from build123d import *

# Parameters (mm, degrees)
CSK_FOR_M3_FLAT_HEAD_MACHINE_SCREW1_AT_2_COUNT = 2
CSK_FOR_M3_FLAT_HEAD_MACHINE_SCREW1_AT_2_PITCH = 13.856406461
CSK_FOR_M3_FLAT_HEAD_MACHINE_SCREW1_AT_3_COUNT = 2
CSK_FOR_M3_FLAT_HEAD_MACHINE_SCREW1_AT_3_PITCH = 13.856406461


with BuildPart() as part:
    # Esquisse1 → Révolution1 (revolve)
    with BuildSketch(Plane.XY, mode=Mode.PRIVATE) as r_volution1_sk:
        Polygon((3, -3.2), (3, 3.2), (6, 3.2), (6, 2), (4.5, 2), (4.5, -1), (11.5, -1), (11.5, -3.2), align=None)
    revolve(r_volution1_sk.sketch.rotate(Axis((0, 4.689873418, 0), (0, -1, 0)), 90), axis=Axis((0, 4.689873418, 0), (0, -1, 0)))

    # Esquisse4 → CSK for M3 Flat Head Machine Screw1 (revolve, cut)
    with BuildSketch(Plane(origin=(-6.92820323, -1, 4), x_dir=(0, 0, 1), z_dir=(1, 0, 0))):
        Polygon((0, 0), (0, 2.2), (1.7, 2.2), (1.7, 1.05), (2.75, 0), align=None)
    csk_for_m3_flat_head_machine_screw1 = revolve(axis=Axis((-6.92820323, 5.35, 4), (0, -1, 0)), mode=Mode.SUBTRACT)

    # CSK for M3 Flat Head Machine Screw1 at 2: CSK for M3 Flat Head Machine Screw1 ×2
    with Locations(*[(i * CSK_FOR_M3_FLAT_HEAD_MACHINE_SCREW1_AT_2_PITCH, 0, 0) for i in range(1, CSK_FOR_M3_FLAT_HEAD_MACHINE_SCREW1_AT_2_COUNT)]):
        add(csk_for_m3_flat_head_machine_screw1, mode=Mode.SUBTRACT)

    # CSK for M3 Flat Head Machine Screw1 at 3: CSK for M3 Flat Head Machine Screw1 ×2
    with Locations(*[Vector(0.5000000000000041, 0, -0.8660254037844364) * (i * CSK_FOR_M3_FLAT_HEAD_MACHINE_SCREW1_AT_3_PITCH) for i in range(1, CSK_FOR_M3_FLAT_HEAD_MACHINE_SCREW1_AT_3_COUNT)]):
        add(csk_for_m3_flat_head_machine_screw1, mode=Mode.SUBTRACT)


solid = part.part
Could you check a few things on this model? Use its own coordinates, in mm. A direction names the side the tool comes from. Give positions to 0.01 mm unless a question says otherwise; leave off trailing zeros. Write each loop counter-clockwise with the first axis right and the second up, starting at its lowest first coordinate (ties: lowest second). Pieces come first, ordered by that corner, then holes. Notation, with made-up numbers: (83, 85) -> (87, 85) arc R26 ccw to (87, 123) -> close; hole circle Ø5 at (77, 12.5). An arc over 180 degrees is marked (long way). Answer as a JSON object with one key per item and string values.
Q1. Suppose I cut it at A-A on z = 0. Write out the boundary of the cut face in (x, y).
Taken from the geometry:
{"outline": "(-11.5, -3.2) -> (-3, -3.2) -> (-3, 3.2) -> (-6, 3.2) -> (-6, 2) -> (-4.5, 2) -> (-4.5, -1) -> (-11.5, -1) -> close; (3, -3.2) -> (11.5, -3.2) -> (11.5, -1) -> (4.5, -1) -> (4.5, 2) -> (6, 2) -> (6, 3.2) -> (3, 3.2) -> close"}
Q2. Suppose I cut it at B-B on x = 0. Write out the boundary of the cut face in (y, z).
Taken from the geometry:
{"outline": "(-3.2, -11.5) -> (-1, -11.5) -> (-1, -10.75) -> (-2.05, -9.7) -> (-3.2, -9.7) -> close; (-3.2, -6.3) -> (-2.05, -6.3) -> (-1, -5.25) -> (-1, -4.5) -> (2, -4.5) -> (2, -6) -> (3.2, -6) -> (3.2, -3) -> (-3.2, -3) -> close; (-3.2, 3) -> (3.2, 3) -> (3.2, 6) -> (2, 6) -> (2, 4.5) -> (-1, 4.5) -> (-1, 11.5) -> (-3.2, 11.5) -> close"}
Q3. Suppose I cut it at D-D on y = 1. Write out the boundary of the cut face in (x, z).
Taken from the geometry:
{"outline": "circle Ø9 at (0, 0); hole circle Ø6 at (0, 0)"}
Q4. We'd pull the mould along X, two halves only. Please class faces 3 (the cylindrical face through (-6.28, -2.62, 5.57)), 4 (the cylindrical face through (-1.15, -2.62, -9.25)), 5 (the cylindrical face through (-1.802, 2.592, 5.723)), 6 (the flat face through (2.4, -3.2, 2.4)): released by +X, released by -X, zero draft, split by the parting line, or undercut.
Taken from the geometry:
{"face 3": "undercut", "face 4": "undercut", "face 5": "split by the parting line", "face 6": "zero draft"}
Q5. Will these pins go through, and if not, where does the flat tip stop? pin 1 Ø3 at (x, y) = (-7, -2) entering from -Z; pin 2 Ø4 at (x, z) = (8.5, 6) entering from +Y; pin 3 Ø1 at (y, z) = (2.5, 0.5) entering from +X.
Taken from the geometry:
{"pin 1": "stops at z = -10.1", "pin 2": "stops at y = -1", "pin 3": "stops at x = 6"}
Q6. Which directions (+Z, -Z, +X, -X, +Y, -Y) give clear straight access to the entire face, cutting with the end or side of a thin tool? Please do faces 1 (the flat face through (0, -1, -5)), 2 (the cylindrical face through (7.58, -2.62, 5.57)).
Taken from the geometry:
{"face 1": "none", "face 2": "+Y, -Y"}
Q7. Suppose I cut it at C-C on z = 4. Write out the boundary of the cut face in (x, y).
Taken from the geometry:
{"outline": "(-10.78, -3.2) -> (-8.63, -3.2) -> (-8.63, -2.05) -> (-9.68, -1) -> (-10.78, -1) -> close; (-5.23, -3.2) -> (5.23, -3.2) -> (5.23, -2.05) -> (4.18, -1) -> (2.06, -1) -> (2.06, 2) -> (4.47, 2) -> (4.47, 3.2) -> (-4.47, 3.2) -> (-4.47, 2) -> (-2.06, 2) -> (-2.06, -1) -> (-4.18, -1) -> (-5.23, -2.05) -> close; (8.63, -3.2) -> (10.78, -3.2) -> (10.78, -1) -> (9.68, -1) -> (8.63, -2.05) -> close"}
Q8. Please list where these lines run through material, in increasing order: L1, parallel to X at y = -2.5, z = 4; L2, parallel to Y at x = 4.5, z = -3.75; L3, parallel to X at y = 0, z = 0.
Taken from the geometry:
{"L1": "x = -10.78 to -8.63, -5.23 to 5.23, 8.63 to 10.78", "L2": "y = -3.2 to -1, 2 to 3.2", "L3": "x = -4.5 to -3, 3 to 4.5"}
